from build123d import *

# Parameters (mm, degrees)
F0_W     = 50
F0_H     = 50
F2_DEPTH = 5
F1_R     = 4
F1_R_2   = 1.35
F1_R_3   = 5
F1_R_4   = 1.4
F3_DEPTH = 6
F1_R_5   = 1.45
F1_R_6   = 1.5
F4_DEPTH = 10
F1_R_7   = 1.55
F1_R_8   = 1.6
F5_DEPTH = 12


with BuildPart() as f2:
    # F0 (on Front) → F2 (new body)
    with BuildSketch(Plane.XZ):
        Rectangle(F0_W, F0_H)
    extrude(amount=-F2_DEPTH)

    # F1 (on Front) → F3 (join)
    with BuildSketch(Plane.XZ):
        with Locations((-18.170596, 15.871764)):
            Circle(F1_R)
        with Locations((-18.170596, 15.871764)):
            Circle(F1_R_2, mode=Mode.SUBTRACT)
        with Locations((-6.920179, 15.756146)):
            Circle(F1_R_3)
        with Locations((-6.920179, 15.756146)):
            Circle(F1_R_2, mode=Mode.SUBTRACT)
        with Locations((6.124761, 15.85988)):
            Circle(F1_R)
        with Locations((6.124761, 15.85988)):
            Circle(F1_R_4, mode=Mode.SUBTRACT)
        with Locations((18.083698, 15.717511)):
            Circle(F1_R_3)
        with Locations((18.083698, 15.717511)):
            Circle(F1_R_4, mode=Mode.SUBTRACT)
    extrude(amount=F3_DEPTH)

    # F1 (on Front) → F4 (join)
    with BuildSketch(Plane.XZ):
        with Locations((-18.362585, 1.053578)):
            Circle(F1_R)
        with Locations((-18.362585, 1.053578)):
            Circle(F1_R_5, mode=Mode.SUBTRACT)
        with Locations((-6.830752, 0.341737)):
            Circle(F1_R_3)
        with Locations((-6.830752, 0.341737)):
            Circle(F1_R_5, mode=Mode.SUBTRACT)
        with Locations((7.406075, 0.341737)):
            Circle(F1_R)
        with Locations((7.406075, 0.341737)):
            Circle(F1_R_6, mode=Mode.SUBTRACT)
        with Locations((18.795539, -0.085368)):
            Circle(F1_R_3)
        with Locations((18.795539, -0.085368)):
            Circle(F1_R_6, mode=Mode.SUBTRACT)
    extrude(amount=F4_DEPTH)

    # F1 (on Front) → F5 (join)
    with BuildSketch(Plane.XZ):
        with Locations((-6.889718, -15.475452)):
            Circle(F1_R_3)
        with Locations((-6.889718, -15.475452)):
            Circle(F1_R_7, mode=Mode.SUBTRACT)
        with Locations((-18.220215, -15.475452)):
            Circle(F1_R)
        with Locations((-18.220215, -15.475452)):
            Circle(F1_R_7, mode=Mode.SUBTRACT)
        with Locations((6.124761, -15.475452)):
            Circle(F1_R)
        with Locations((6.124761, -15.475452)):
            Circle(F1_R_8, mode=Mode.SUBTRACT)
        with Locations((17.798963, -15.475452)):
            Circle(F1_R_3)
        with Locations((17.798963, -15.475452)):
            Circle(F1_R_8, mode=Mode.SUBTRACT)
    extrude(amount=F5_DEPTH)


solid = f2.part
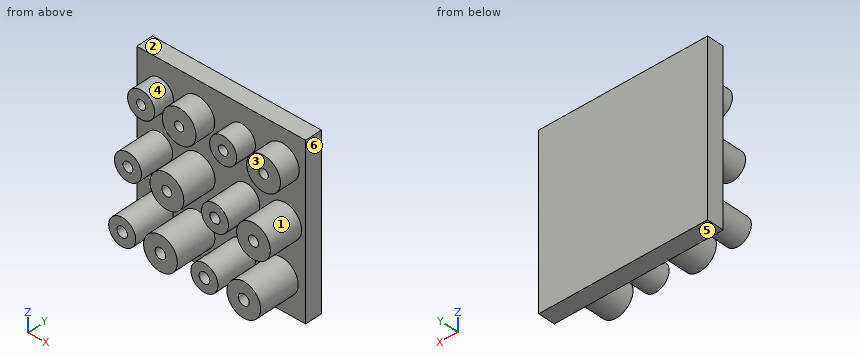
Model file for the job. Use its own axes, mm. Face numbers are marked on the shaded views. A direction names the side the tool comes from. Round coordinates to 2 decimals unless told otherwise and drop trailing zeros. Loops run counter-clockwise (first coordinate to the right, second up) from the corner with the lowest first, then second, coordinate; pieces in that order, holes last. Notation, with made-up numbers: (3, -1) -> (26, -1) arc R5 cw to (26, 7) -> close; hole circle Ø7 at (-27, 31). An arc over 180 degrees is marked (long way). Answer as CSV lines item,"result". Start each with the question number.
1) Pin check, flat tips, straight feed: P1, Ø3, axis at x = 17.5, z = -1, coming from the -Y side; P2, Ø3.5, axis at x = -6.92, z = 15.76, coming from the -Y side; P3, Ø1, axis at x = -10.5, z = 9, coming from the -Y side; P4, Ø5, axis at x = -18.22, z = -15.48, coming from the -Y side. Stop position of each tip, or through.
2) Slice it at C-C (z = -22). List the corners of the cut face in (x, y).
3) Tool access for the marked faces 1, 2 and 3: list every direction of +Z, -Z, +X, -X, +Y, -Y with a clear straight run to the whole face (end or side of a thin tool).
4) Slice it at B-B (y = -11). List the corners of the cut face in (x, z), plus the area to 3 significant figures.
5) Slice it at A-A (y = -5.25). State how many separate pieces and enclosed holes the cut face has, plus the area to 3 significant figures.
6) Mould opens along X. For the marked faces 4, 5 and 6 say: +X half, -X half, draft (parallel to the pull), parting line (faces both ways), or undercut.
7) Slice it at D-D (x = 21.5). List the corners of the cut face in (y, z), plus the area to 3 significant figures.
8) Probe line 1 along Z through (x, y) = (14.5, -1); line 2 along Z through (x, y) = (5, -6.5); line 3 along Y through (x, z) = (23.5, 3). List the from-to ranges inside material, lowest first.
Filled in:
1,P1,"stops at y = -10"
1,P2,"stops at y = -6"
1,P3,"stops at y = 0"
1,P4,"stops at y = -12"
2,outline,"(-25, 0) -> (25, 0) -> (25, 5) -> (-25, 5) -> close"
3,face 1,"-Y"
3,face 2,"+Z, +X, -X, +Y, -Y"
3,face 3,"+Z, +X, -X, -Y"
4,outline,"circle Ø8 at (-18.22, -15.48); circle Ø10 at (-6.89, -15.48); circle Ø8 at (6.12, -15.48); circle Ø10 at (17.8, -15.48); hole circle Ø3.1 at (-18.22, -15.48); hole circle Ø3.1 at (-6.89, -15.48); hole circle Ø3.2 at (6.12, -15.48); hole circle Ø3.2 at (17.8, -15.48)"
4,area,"226 mm2"
5,separate pieces,"12"
5,enclosed holes,"12"
5,area,"691 mm2"
6,face 4,"undercut"
6,face 5,"draft"
6,face 6,"+X half"
7,outline,"(-12, -18.84) -> (0, -18.84) -> (0, -25) -> (5, -25) -> (5, 25) -> (0, 25) -> (0, 19.37) -> (-6, 19.37) -> (-6, 12.07) -> (0, 12.07) -> (0, 4.12) -> (-10, 4.12) -> (-10, -4.29) -> (0, -4.29) -> (0, -12.11) -> (-12, -12.11) -> close"
7,area,"459 mm2"
8,line 1,"z = -19.23 to -11.72, -2.64 to 2.47, 12.23 to 19.2"
8,line 2,"z = -19.31 to -16.61, -14.34 to -11.64, -2.85 to 3.54"
8,line 3,"y = 0 to 5"
